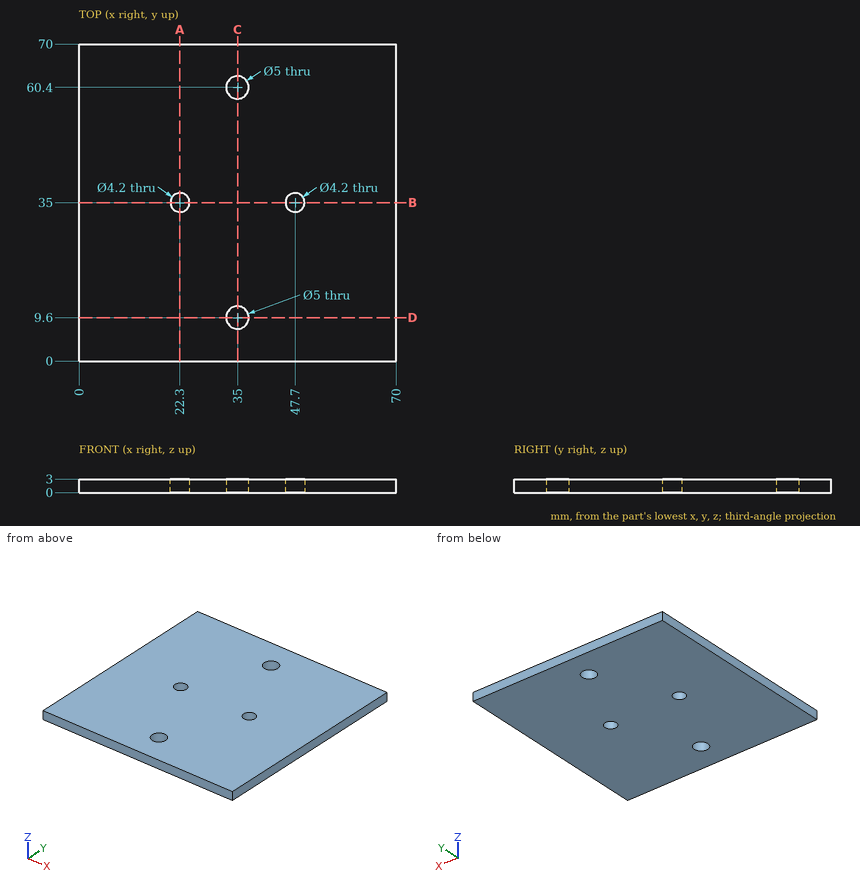
Source: three-view drawing plus pictorial views. Frame: mm from the lowest corner of the part. Round coordinates to 2 decimals unless told otherwise and drop trailing zeros. Loops run counter-clockwise (first coordinate to the right, second up) from the corner with the lowest first, then second, coordinate; pieces in that order, holes last.
Item 1: Section D-D, the plane y = 9.6. Output: boundary loops of the cut face in (x, z), plus the area to 3 significant figures.
Checked values:
outline: (0, 0) - (32.5, 0) - (32.5, 3) - (0, 3) - close; (37.5, 0) - (70, 0) - (70, 3) - (37.5, 3) - close
area: 195 mm2
Item 2: Section A-A, the plane x = 22.3. Output: boundary loops of the cut face in (y, z).
Checked values:
outline: (0, 0) - (32.9, 0) - (32.9, 3) - (0, 3) - close; (37.1, 0) - (70, 0) - (70, 3) - (37.1, 3) - close
Item 3: Section C-C, the plane x = 35. Output: boundary loops of the cut face in (y, z).
Checked values:
outline: (0, 0) - (7.1, 0) - (7.1, 3) - (0, 3) - close; (12.1, 0) - (57.9, 0) - (57.9, 3) - (12.1, 3) - close; (62.9, 0) - (70, 0) - (70, 3) - (62.9, 3) - close
Item 4: Line query: L1, parallel to Y at x = 35, z = 1.4; L2, parallel to Y at x = 47.7, z = 1; L3, parallel to X at y = 34.5, z = 2.35. Output: solid intervals per line, ascending.
Checked values:
L1: y = 0 to 7.1, 12.1 to 57.9, 62.9 to 70
L2: y = 0 to 32.9, 37.1 to 70
L3: x = 0 to 20.26, 24.34 to 45.66, 49.74 to 70
Item 5: Section B-B, the plane y = 35. Output: boundary loops of the cut face in (x, z), plus the area to 3 significant figures.
Checked values:
outline: (0, 0) - (20.2, 0) - (20.2, 3) - (0, 3) - close; (24.4, 0) - (45.6, 0) - (45.6, 3) - (24.4, 3) - close; (49.8, 0) - (70, 0) - (70, 3) - (49.8, 3) - close
area: 185 mm2
